Source: three-view drawing plus pictorial views. Frame: mm from the lowest corner of the part. A direction names the side the tool comes from. Give positions to 0.01 mm unless a question says otherwise; leave off trailing zeros. Order: outer loops, then holes, each group sorted by start corner. A loop starts at its lowest first (then second) coordinate and runs counter-clockwise, first axis right, second up.
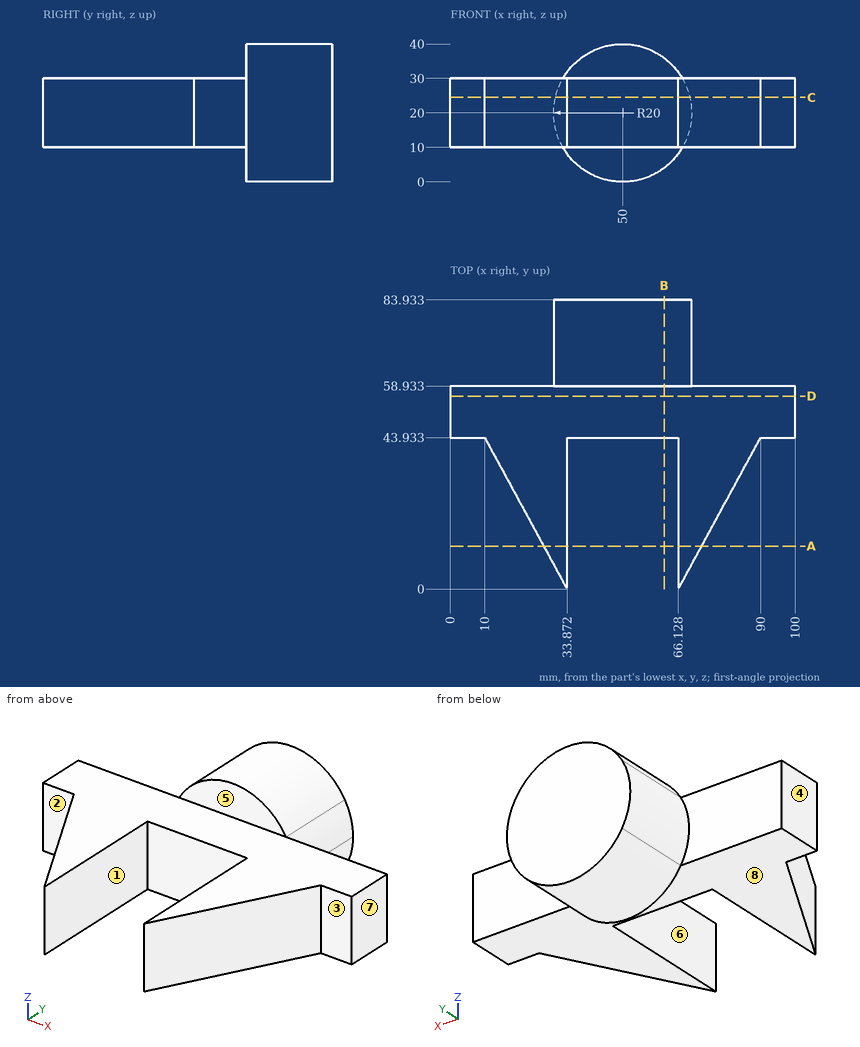
1) Section query A-A on y = 12.5. Output: boundary loops of the cut face in (x, z).
Checks:
outline: (27.08, 10) - (33.87, 10) - (33.87, 30) - (27.08, 30) - close; (66.13, 10) - (72.92, 10) - (72.92, 30) - (66.13, 30) - close
2) Pull-direction query (X, two-part tool) for the marked faces 6, 7 and 8; classes: +X half, -X half, draft (parallel to the pull), parting line (faces both ways), or undercut.
Checks:
face 6: undercut
face 7: +X half
face 8: draft
3) Reachability of the marked faces 1, 2, 3, 4 and 5 from +Z, -Z, +X, -X, +Y, -Y: full face, straight path, thin tool, end or side. Return the list, or none.
Checks:
face 1: +Z, -Z, -Y
face 2: +Z, -Z, -X, -Y
face 3: +Z, -Z, +X, -Y
face 4: +Z, -Z, -X, +Y, -Y
face 5: +Z, +X, -X, -Y
4) Section query C-C on z = 24.5. Output: boundary loops of the cut face in (x, y), and give its area (3 significant figures).
Checks:
outline: (0, 43.93) - (10, 43.93) - (33.87, 0) - (33.87, 43.93) - (66.13, 43.93) - (66.13, 0) - (90, 43.93) - (100, 43.93) - (100, 58.93) - (69.49, 58.93) - (69.49, 83.93) - (30.51, 83.93) - (30.51, 58.93) - (0, 58.93) - close
area: 3,520 mm2
5) First-contact query: pin 1 Ø8 at (x, z) = (81, 29.5) entering from -Y; pin 2 Ø16 at (y, z) = (21, 24) entering from +X (1 decimal); pin 3 Ø4 at (x, z) = (88, 9) entering from +Y. Flat tips, straight axial feed; report the tip coordinate or a pass-through.
Checks:
pin 1: stops at y = 20.01
pin 2: stops at x = 81.9
pin 3: stops at y = 58.93
6) Ray query, L1, parallel to Y at x = 58, z = 18.5; L2, parallel to Z at x = 25, y = 35.5; L3, parallel to Y at x = 9.5, z = 13.5. Return the intervals inside material, ascending.
Checks:
L1: y = 43.93 to 83.93
L2: z = 10 to 30
L3: y = 43.93 to 58.93
7) Section query B-B on x = 62. Output: boundary loops of the cut face in (y, z).
Checks:
outline: (43.93, 10) - (58.93, 10) - (58.93, 4) - (83.93, 4) - (83.93, 36) - (58.93, 36) - (58.93, 30) - (43.93, 30) - close
8) Section query D-D on y = 56. Output: boundary loops of the cut face in (x, z), and give its area (3 significant figures).
Checks:
outline: (0, 10) - (100, 10) - (100, 30) - (0, 30) - close
area: 2,000 mm2
